Drawing for the job (mm, zero at the part's lowest x, y, z). A direction names the side the tool comes from. Give positions to 0.01 mm unless a question says otherwise; leave off trailing zeros. Write each loop counter-clockwise with the first axis right and the second up, starting at its lowest first coordinate (ties: lowest second). Pieces come first, ordered by that corner, then holes. Notation, with made-up numbers: M 41,-27.5 L 82,-27.5 A14 cw 82,-13.5 Z; hole C 88.25,79.25 d4. An arc over 180 degrees is marked long. Use a Markdown table: item, result. Add a question column.
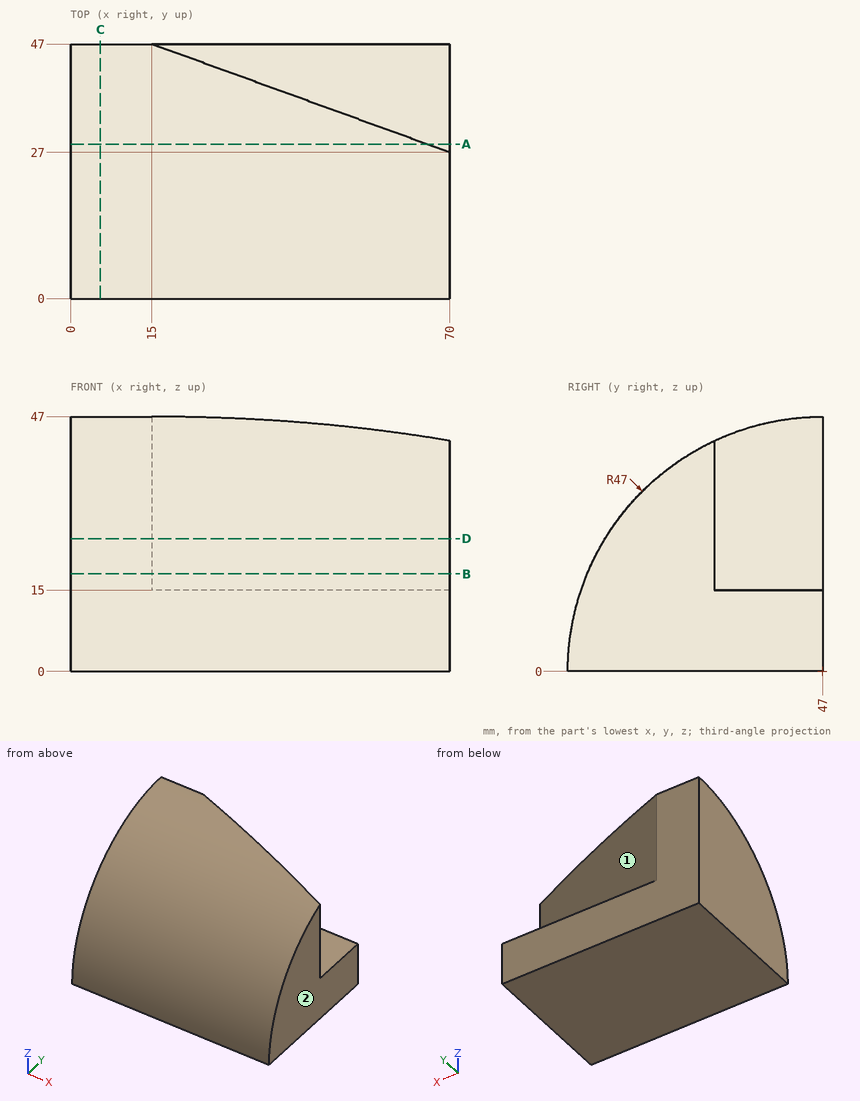
1. Tool access for the marked faces 1 and 2: list every direction of +Z, -Z, +X, -X, +Y, -Y with a clear straight run to the whole face (end or side of a thin tool).
2. Cut at C-C (x = 5.5). Write the cut outline in (y, z).
3. Cut at A-A (y = 28.5). Write the cut outline in (x, z) (3 decimals).
4. Cut at B-B (z = 18). Write the cut outline in (x, y), then the cut area to 3 significant figures.
5. Flat gauge pins, fed straight in: pin 1 (2 mm diameter, centred on x = 37, z = 28.5, fed in from -Y); pin 2 (5 mm diameter, centred on x = 13.5, y = 20, fed in from +Z); pin 3 (1.5 mm diameter, centred on x = 13.5, y = 30.5, fed in from +Z); pin 4 (12 mm diameter, centred on y = 32.5, z = 34.5, fed in from -X). Where does each tip first touch, or does it go through?
6. Cut at D-D (z = 24.5). Write the cut outline in (x, y), then the cut area to 3 significant figures.
7. Drill centre lines: probe 1 along Z at (x, y) = (37, 38); probe 2 along Y at (x, z) = (65.5, 32); probe 3 along Y at (x, z) = (10.5, 9). Where is each one in solid material? Low to high. Write a range as [from, to].
A:
| question | item | result |
|---|---|---|
| 1 | face 1 | +Z, +X, +Y |
| 1 | face 2 | +Z, -Z, +X, +Y, -Y |
| 2 | outline | M 0,0 L 47,0 L 47,47 A47 ccw Z |
| 3 | outline | M 0,0 L 70,0 L 70,15 L 65.875,15 L 65.875,43.206 L 0,43.206 Z |
| 4 | outline | M 0,3.58 L 70,3.58 L 70,27 L 15,47 L 0,47 Z |
| 4 | area | 2,490 mm² |
| 5 | pin 1 | stops at y = 8.89 |
| 5 | pin 2 | stops at z = 40.11 |
| 5 | pin 3 | stops at z = 44.28 |
| 5 | pin 4 | stops at x = 0 |
| 6 | outline | M 0,6.89 L 70,6.89 L 70,27 L 15,47 L 0,47 Z |
| 6 | area | 2,260 mm² |
| 7 | probe 1 | z = [0, 46.13] |
| 7 | probe 2 | y = [12.58, 28.64] |
| 7 | probe 3 | y = [0.87, 47] |
